```python
from build123d import *

# Parameters (mm, degrees)
BOSS_EXTRUDE1_DEPTH = 228.6
SKETCH19_R          = 5.588
CUT_EXTRUDE2_DEPTH  = 235.36596615


with BuildPart() as part:
    # Sketch18 → Boss-Extrude1 (new, symmetric)
    with BuildSketch(Plane(origin=(0, 0, 0), x_dir=(1, 0, 0), z_dir=(0, 1, 0))):
        Polygon((-3.489230953, 38.072508354), (2.664141329, 3.175), (38.1, 3.175), (38.1, 0), (0, 0), (-6.615995569, 37.52117539), align=None)
    extrude(amount=BOSS_EXTRUDE1_DEPTH, both=True)

    # Sketch19 → Cut-Extrude2 (cut, through all)
    with BuildSketch(Plane(origin=(0, 0, -3.175), x_dir=(-1, 0, 0), z_dir=(0, 0, -1))):
        with Locations((-20.382070664, 203.2)):
            Circle(SKETCH19_R)
    cut_extrude2 = extrude(amount=-CUT_EXTRUDE2_DEPTH, mode=Mode.SUBTRACT)

    # Mirror1: Cut-Extrude2 across plane
    add(cut_extrude2.mirror(Plane.ZX), mode=Mode.SUBTRACT)


solid = part.part
```
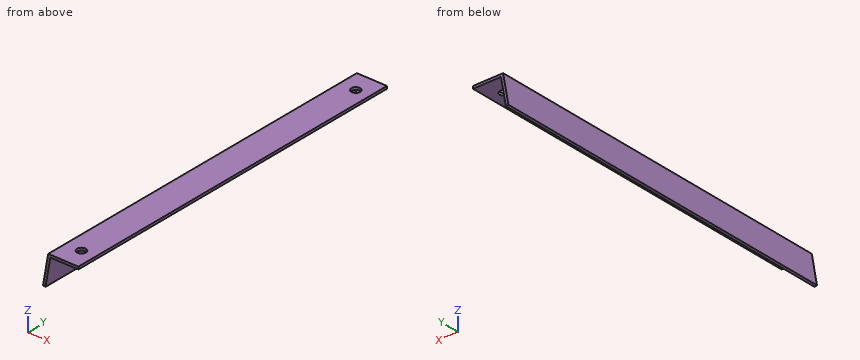
Source: CAD feature listing. Evaluate the final solid. Frame: model axes, mm. Round coordinates to 2 decimals unless told otherwise and drop trailing zeros. Loops run counter-clockwise (first coordinate to the right, second up) from the corner with the lowest first, then second, coordinate; pieces in that order, holes last. Notation, with made-up numbers: M 47,16 L 104,16 A22 cw 104,51 Z; hole C 1.25,58.5 d2. An arc over 180 degrees is marked long. Use a Markdown table: item, result. Add a question column.
1. Cut plane D-D, the plane z = -9. Output: boundary loops of the cut face in (x, y), and give its area (3 significant figures).
2. Cut plane B-B, the plane y = 125.5. Output: boundary loops of the cut face in (x, z) (1 decimal), and give its area (3 significant figures).
3. Cut plane A-A, the plane y = -203.2. Output: boundary loops of the cut face in (x, z) (1 decimal).
4. Contact query for flat-ended pins moving along their axis: pin 1 (10 mm diameter, centred on y = 142.5, z = -13, fed in from +X); pin 2 (2 mm diameter, centred on x = 31.5, y = -68, fed in from -Z) (3 decimals); pin 3 (3 mm diameter, centred on y = -61.5, z = -18, fed in from +X). Output: stop coordinate, or through.
5. Ray query, line 1 along Z through (x, y) = (19.5, 45.5) (3 decimals); line 2 along X through (y, z) = (-203, -1); line 3 along X through (y, z) = (-141, -9). Return the intervals inside material, ascending. Write a range as [from, to].
6. Cut plane C-C, the plane x = 7.5. Output: boundary loops of the cut face in (y, z) (3 decimals), and give its area (3 significant figures).
Solution:
| question | item | result |
|---|---|---|
| 1 | outline | M -1.59,-228.6 L 1.64,-228.6 L 1.64,228.6 L -1.59,228.6 Z |
| 1 | area | 1,470 mm2 |
| 2 | outline | M -6.6,-37.5 L -3.5,-38.1 L 2.7,-3.2 L 38.1,-3.2 L 38.1,0 L 0,0 Z |
| 2 | area | 233 mm2 |
| 3 | outline | M -6.6,-37.5 L -3.5,-38.1 L 2.7,-3.2 L 14.8,-3.2 L 14.8,0 L 0,0 Z; M 26,-3.2 L 38.1,-3.2 L 38.1,0 L 26,0 Z |
| 4 | pin 1 | stops at x = 1.81 |
| 4 | pin 2 | stops at z = -3.175 |
| 4 | pin 3 | stops at x = 0.31 |
| 5 | line 1 | z = [-3.175, 0] |
| 5 | line 2 | x = [-0.18, 14.8], [25.97, 38.1] |
| 5 | line 3 | x = [-1.59, 1.64] |
| 6 | outline | M -228.6,-3.175 L 228.6,-3.175 L 228.6,0 L -228.6,0 Z |
| 6 | area | 1,450 mm2 |
